Build history of the part. All positions in model axes, mm. Round coordinates to 2 decimals unless told otherwise and drop trailing zeros. Write each loop counter-clockwise with the first axis right and the second up, starting at its lowest first coordinate (ties: lowest second). Pieces come first, ordered by that corner, then holes. Notation, with made-up numbers: (6, 12) -> (40, 12) arc R17 ccw to (40, 39) -> close; hole circle Ø2 at (76, 74). An arc over 180 degrees is marked (long way). Return JSON: item names as keys, results as strings.
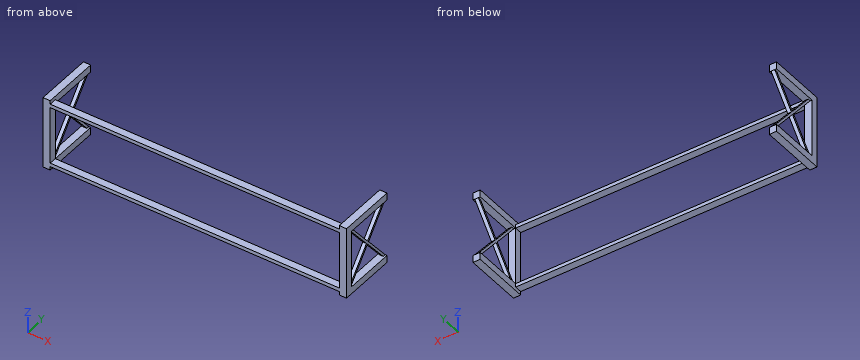
from build123d import *

# Parameters (mm, degrees)
BOSS_EXTRUDE1_DEPTH = 5
BOSS_EXTRUDE2_DEPTH = 2.5
SKETCH2_W           = 200
SKETCH2_H           = 5
BOSS_EXTRUDE3_DEPTH = 10


with BuildPart() as part:
    # Sketch1 → Boss-Extrude1 (new body, symmetric)
    with BuildSketch(Plane(origin=(0, 0, 0), x_dir=(0, 0, -1), z_dir=(1, 0, 0))):
        Polygon((50, 0), (-50, 0), (-50, 80), (-40, 80), (-40, 10), (40, 10), (40, 80), (50, 80), align=None)
    extrude(amount=BOSS_EXTRUDE1_DEPTH, both=True)

    # Sketch1_4 → Boss-Extrude2 (add, symmetric)
    with BuildSketch(Plane(origin=(0, 0, 0), x_dir=(0, 0, -1), z_dir=(1, 0, 0))):
        Polygon((0, 47.12132), (-40, 80), (-40, 76.135024964), (-2.12132, 45), (-40, 13.864975036), (-40, 10), (0, 42.87868), (0, 45), align=None)
        Polygon((40, 80), (0, 47.12132), (0, 45), (0, 42.87868), (40, 10), (40, 13.864975036), (2.12132, 45), (40, 76.135024964), align=None)
    extrude(amount=BOSS_EXTRUDE2_DEPTH, both=True)

    # Sketch2 → Boss-Extrude3 (add)
    with BuildSketch(Plane(origin=(0, 0, 0), x_dir=(1, 0, 0), z_dir=(0, 1, 0))):
        with Locations((105, 42.5)):
            Rectangle(SKETCH2_W, SKETCH2_H)
        with Locations((105, -42.5)):
            Rectangle(SKETCH2_W, SKETCH2_H)
    extrude(amount=BOSS_EXTRUDE3_DEPTH)

    # Mirror1: part across plane


with BuildPart() as part_1:
    add(part.part)
    add(part.part.mirror(Plane(origin=(205, 10, 40), x_dir=(0, 0, 1), z_dir=(-1, 0, 0))))


solid = part_1.part
Q1. Saw through at A-A on x = 181.5. List the corners of the cut face in (y, z).
Verdict:
{"outline": "(0, -45) -> (10, -45) -> (10, -40) -> (0, -40) -> close; (0, 40) -> (10, 40) -> (10, 45) -> (0, 45) -> close"}
Q2. Pin check, flat tips, straight feed: pin 1 Ø6 at (y, z) = (23, -38.5) entering from +X; pin 2 Ø8 at (x, y) = (221.5, 3.5) entering from -Z; pin 3 Ø2.5 at (x, z) = (118, -41.5) entering from +Y; pin 4 Ø5 at (x, y) = (273, 6.5) entering from +Z. Stop position of each tip, or through.
Verdict:
{"pin 1": "stops at x = 415", "pin 2": "stops at z = -45", "pin 3": "stops at y = 10", "pin 4": "stops at z = 45"}
Q3. Saw through at B-B on z = 13. List the corners of the cut face in (x, y), then the cut area to 3 significant figures.
Verdict:
{"outline": "(-5, 0) -> (5, 0) -> (5, 10) -> (-5, 10) -> close; (-2.5, 32.19) -> (2.5, 32.19) -> (2.5, 36.06) -> (-2.5, 36.06) -> close; (-2.5, 53.94) -> (2.5, 53.94) -> (2.5, 57.81) -> (-2.5, 57.81) -> close; (405, 0) -> (415, 0) -> (415, 10) -> (405, 10) -> close; (407.5, 32.19) -> (412.5, 32.19) -> (412.5, 36.06) -> (407.5, 36.06) -> close; (407.5, 53.94) -> (412.5, 53.94) -> (412.5, 57.81) -> (407.5, 57.81) -> close", "area": "277 mm²"}
Q4. Wall check: L1, parallel to X at y = 5, z = 14.5; L2, parallel to X at y = 31.5, z = 17; L3, parallel to Y at x = 309, z = -43. Give the ranges that are in metal, low to high.
Verdict:
{"L1": "x = -5 to 5, 405 to 415", "L2": "x = -2.5 to 2.5, 407.5 to 412.5", "L3": "y = 0 to 10"}
Q5. Saw through at C-C on y = 22. Count the separate pieces of the cut face and the enclosed holes in it, then the cut area to 3 significant figures.
Verdict:
{"separate pieces": "8", "enclosed holes": "0", "area": "494 mm²"}
